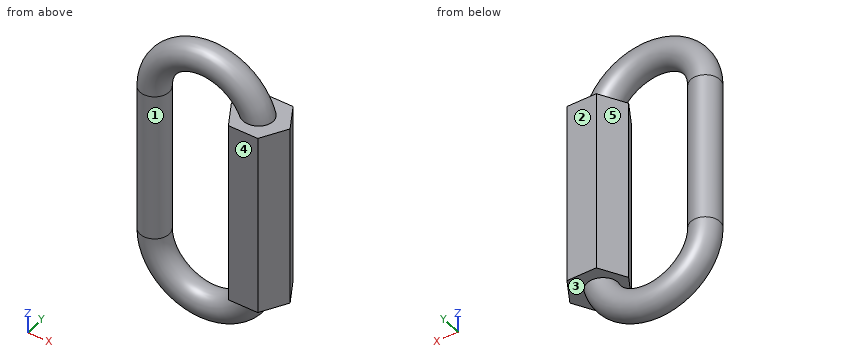
```python
from build123d import *

# Parameters (mm, degrees)
SKETCH1_R                = 2.53
BOSS_EXTRUDE1_DEPTH      = 16
BOSS_EXTRUDE1_DEPTH_BACK = 16


with BuildPart() as part:
    # Sweep1: sweep along a path in Sketch2
    with BuildLine(Plane(origin=(0, 0, 0), x_dir=(1, 0, 0), z_dir=(0, 1, 0))) as sweep1_path:
        Line((0, -13.05), (0, 13.05))
        ThreePointArc((0, 13.05), (-9.235, 22.285), (-18.47, 13.05))
        Line((-18.47, 13.05), (-18.47, -13.05))
        ThreePointArc((-18.47, -13.05), (-9.235, -22.285), (0, -13.05))
    # Sketch1 → Sweep1 (sweep)
    with BuildSketch(Plane.XY):
        Circle(SKETCH1_R)
    sweep(path=sweep1_path.line)

    # Sketch3 → Boss-Extrude1 (add, two sides)
    with BuildSketch(Plane.XY) as boss_extrude1_sk:
        Polygon((-2.554774941, 4.425), (-5.109549882, 0), (-2.554774941, -4.425), (2.554774941, -4.425), (5.109549882, 0), (2.554774941, 4.425), align=None)
    extrude(amount=BOSS_EXTRUDE1_DEPTH)
    extrude(boss_extrude1_sk.sketch, amount=-BOSS_EXTRUDE1_DEPTH_BACK)


solid = part.part
```
Verification items for the finished model (mm, model axes). Face numbers are marked on the shaded views. A direction names the side the tool comes from. Round coordinates to 2 decimals unless told otherwise and drop trailing zeros. Order: outer loops, then holes, each group sorted by start corner. A loop starts at its lowest first (then second) coordinate and runs counter-clockwise, first axis right, second up.
1) Cross-section at A-A, the plane z = -11. Record the cut outline in (x, y) (3 decimals).
Geometry says:
outline: circle Ø5.06 at (-18.47, 0); (-5.11, 0) - (-2.555, -4.425) - (2.555, -4.425) - (5.11, 0) - (2.555, 4.425) - (-2.555, 4.425) - close
2) Cross-section at C-C, the plane y = -1.5. Record the cut outline in (x, z) (3 decimals), plus the area to 3 significant figures.
Geometry says:
outline: (-20.507, -13.05) arc R11.272 ccw to (1.645, -16) - (4.244, -16) - (4.244, 16) - (1.645, 16) arc R11.272 ccw to (-20.507, 13.05) - close; hole (-16.433, -13.05) arc R7.198 ccw to (-2.67, -16) - (-4.244, -16) - (-4.244, 16) - (-2.67, 16) arc R7.198 ccw to (-16.433, 13.05) - close
area: 590 mm2
3) Material ranges on line 1 (Z direction, x = -3.25, y = -0.5); line 2 (Z direction, x = -4.25, y = -1); line 3 (X direction, y = -2, z = -14.5), recorded low to high.
Geometry says:
line 1: z = -23.12 to -16.18, -16 to 16, 16.18 to 23.12
line 2: z = -23.48 to -17.84, -16 to 16, 17.84 to 23.48
line 3: x = -19.92 to -16.78, -3.95 to 3.95
4) Tool access check on the marked faces 3, 4 and 5. Record the directions out of +Z, -Z, +X, -X, +Y, -Y that give a thin tool (end or side, any length) a straight path to the whole face; none if there is none.
Geometry says:
face 3: none
face 4: +Z, -Z, +X, -X, -Y
face 5: +Y
5) Cross-section at B-B, the plane y = 0.5. Record the cut outline in (x, z) (3 decimals).
Geometry says:
outline: (-20.95, -13.05) arc R11.715 ccw to (2.103, -16) - (4.821, -16) - (4.821, 16) - (2.103, 16) arc R11.715 ccw to (-20.95, 13.05) - close; hole (-15.99, -13.05) arc R6.755 ccw to (-3.158, -16) - (-4.821, -16) - (-4.821, 16) - (-3.158, 16) arc R6.755 ccw to (-15.99, 13.05) - close
6) Depth check by flat-ended pin: pin 1 (4 mm diameter, centred on x = -16, y = -2.5, fed in from +Z); pin 2 (1 mm diameter, centred on y = -3.5, z = -1, fed in from +X); pin 3 (2.5 mm diameter, centred on x = 2, y = 0.5, fed in from -Z). Enter the tip coordinate at first touch or a pass-through.
Geometry says:
pin 1: stops at z = 23.25
pin 2: stops at x = 3.38
pin 3: stops at z = -19.21
7) Draft check along Z on the marked faces 1 and 2. Enter one of: +Z half, -Z half, draft (parallel to the pull), parting line (faces both ways), or undercut.
Geometry says:
face 1: undercut
face 2: draft
